from build123d import *

# Parameters (mm, degrees)
SKETCH3_W           = 114.3
SKETCH3_H           = 19.05
BOSS_EXTRUDE1_DEPTH = 3.81
SKETCH4_R           = 13.5453125
BOSS_EXTRUDE2_DEPTH = 9.525
FILLET1_R           = 2.032
SKETCH5_R           = 2.75
CUT_EXTRUDE4_DEPTH  = 12.7


with BuildPart() as part:
    # Sketch3 → Boss-Extrude1 (new body)
    with BuildSketch(Plane(origin=(0, 0, 0), x_dir=(1, 0, 0), z_dir=(0, 1, 0))):
        Rectangle(SKETCH3_W, SKETCH3_H)
    extrude(amount=BOSS_EXTRUDE1_DEPTH)

    # Sketch4 → Boss-Extrude2 (add, symmetric)
    with BuildSketch(Plane.XY):
        with BuildLine():
            Line((-36.071859255, 3.81), (36.071859255, 3.81))
            ThreePointArc((36.071859255, 3.81), (41.198342199, 6.412778013), (42.122274879, 12.087425946))
            ThreePointArc((42.122274879, 12.087425946), (41.806974837, 13.2052175), (41.567140999, 14.341594112))
            Line((41.567140999, 14.341594112), (45.319258538, 15.003193668))
            ThreePointArc((45.319258538, 15.003193668), (67.365546349, 6.979001129), (63.291557028, 30.083742702))
            ThreePointArc((63.291557028, 30.083742702), (61.010906137, 30.694841267), (58.658787305, 30.900625))
            Line((58.658787305, 30.900625), (58.658787305, 34.710625))
            ThreePointArc((58.658787305, 34.710625), (61.672505693, 34.446958806), (64.594653774, 33.663971588))
            ThreePointArc((64.594653774, 33.663971588), (75.750433611, 14.341594112), (58.658787305, 0))
            Line((58.658787305, 0), (-58.658787305, 0))
            ThreePointArc((-58.658787305, 0), (-70.930846463, 5.083253342), (-76.014099805, 17.3553125))
            ThreePointArc((-76.014099805, 17.3553125), (-55.993216901, 34.504703346), (-42.122274879, 12.087425946))
            ThreePointArc((-42.122274879, 12.087425946), (-41.198342199, 6.412778013), (-36.071859255, 3.81))
        make_face()
        with Locations(Location((-58.658787305, 17.3553125, 0), (0, 0, 180))):
            Circle(SKETCH4_R, mode=Mode.SUBTRACT)
    extrude(amount=BOSS_EXTRUDE2_DEPTH, both=True)

    # Fillet1
    # the kernel refuses this fillet: 2.032 mm, written as the material it takes off along each edge
    with BuildSketch(Plane(origin=(58.658787305, 34.710625, 0), x_dir=(0, -1, 0), z_dir=(0, 0, -1)), Plane(origin=(41.567140999, 14.341594112, 0), x_dir=(0.9848077530122078, 0.17364817766693208, 0), z_dir=(0, 0, 1))) as fillet1_piece_1:
        with BuildLine():
            CenterArc((2.16732771, -2.032), FILLET1_R, 90, 97.620348072)
            ThreePointArc((0.153273302, -2.301460275), (0.03836072, -1.153279249), (0, 0))
            Line((0, 0), (2.16732771, 0))
        make_face()
    extrude(amount=15.291396244, mode=Mode.SUBTRACT)
    with BuildSketch(Plane(origin=(58.658787305, 30.900625, 0), x_dir=(0.9978615634411592, -0.06536283505758803, 0), z_dir=(0, 0, -1)), Plane(origin=(45.319258538, 15.003193668, 0), x_dir=(0.23764666877900192, -0.9713516669148425, 0), z_dir=(0, 0, 1))) as fillet1_piece_2:
        with BuildLine():
            CenterArc((1.903537334, -2.027654697), FILLET1_R, 93.747686363, 82.504627273)
            Line((-0.124117363, -1.894837416), (0, 0))
            ThreePointArc((0, 0), (0.885360027, -0.028965791), (1.770720053, 0))
        make_face()
    extrude(amount=14.272245223, mode=Mode.SUBTRACT)
    with BuildSketch(Plane(origin=(45.319258538, 15.003193668, 0), x_dir=(-0.9848077530122076, -0.17364817766693288, 0), z_dir=(0, 0, -1)), Plane(origin=(58.658787305, 30.900625, 0), x_dir=(0, 1, 0), z_dir=(0, 0, 1))) as fillet1_piece_3:
        with BuildLine():
            CenterArc((1.898898089, -2.032), FILLET1_R, 90, 82.504627273)
            ThreePointArc((-0.115739283, -1.766933481), (-0.028965791, -0.885360027), (0, 0))
            Line((0, 0), (1.898898089, 0))
        make_face()
    extrude(amount=14.272245223, mode=Mode.SUBTRACT)
    with BuildSketch(Plane(origin=(41.567140999, 14.341594112, 0), x_dir=(0.23870589854739682, -0.9710919081110089, 0), z_dir=(0, 0, -1)), Plane(origin=(58.658787305, 34.710625, 0), x_dir=(0.9977896842762429, -0.06645107938864023, 0), z_dir=(0, 0, 1))) as fillet1_piece_4:
        with BuildLine():
            CenterArc((2.171529904, -2.027508638), FILLET1_R, 86.189825964, 97.620348072)
            Line((0.144021266, -2.162537232), (0, 0))
            ThreePointArc((0, 0), (1.153279249, 0.03836072), (2.306558498, 0))
        make_face()
    extrude(amount=15.291396244, mode=Mode.SUBTRACT)

    # Sketch5 → Cut-Extrude4 (cut)
    with BuildSketch(Plane(origin=(0, 3.81, 0), x_dir=(1, 0, 0), z_dir=(0, 1, 0))):
        with Locations(Location((-22.225, 0, 0), (0, 0, 270))):
            Circle(SKETCH5_R)
        with Locations(Location((22.225, 0, 0), (0, 0, 270))):
            Circle(SKETCH5_R)
    extrude(amount=-CUT_EXTRUDE4_DEPTH, mode=Mode.SUBTRACT)


solid = part.part
Part model, mm, in its own coordinate system. A direction names the side the tool comes from. Give positions to 0.01 mm unless a question says otherwise; leave off trailing zeros. Order: outer loops, then holes, each group sorted by start corner. A loop starts at its lowest first (then second) coordinate and runs counter-clockwise, first axis right, second up. Notation, with made-up numbers: (26, 83.5) - (41, 83.5) arc R26 cw to (41, 112.5) - close; hole circle Ø11 at (7, 7). An arc over 180 degrees is marked (long way). One line per question, with ' | ' between items.
1. Pull direction X, two halves, no side cores. Call faces 1 (the face through (75.996, 16.567, 0.133)), 2 (the face through (-1, 0, 0)), 3 (the face through (-19.5, 1.93, -0.36)): +X half, -X half, draft (parallel to the pull), parting line (faces both ways), or undercut.
Filled in:
face 1: +X half | face 2: draft | face 3: undercut
2. Band-saw the part on D-D on x = -48. List the corners of the cut face in (y, z) (3 decimals), then the cut area to 3 significant figures.
Filled in:
outline: (0, -9.525) - (8.997, -9.525) - (8.997, 9.525) - (0, 9.525) - close; (25.714, -9.525) - (31.052, -9.525) - (31.052, 9.525) - (25.714, 9.525) - close | area: 273 mm²
3. Band-saw the part on B-B on y = 6.5. List the corners of the cut face in (x, z) (1 decimal).
Filled in:
outline: (-72.2, -9.5) - (-66.8, -9.5) - (-66.8, 9.5) - (-72.2, 9.5) - close; (-50.6, -9.5) - (-41.3, -9.5) - (-41.3, 9.5) - (-50.6, 9.5) - close; (41.3, -9.5) - (50.6, -9.5) - (50.6, 9.5) - (41.3, 9.5) - close; (66.8, -9.5) - (72.2, -9.5) - (72.2, 9.5) - (66.8, 9.5) - close
4. Band-saw the part on C-C on x = -64. List the corners of the cut face in (y, z) (3 decimals), then the cut area to 3 significant figures.
Filled in:
outline: (0.842, -9.525) - (4.908, -9.525) - (4.908, 9.525) - (0.842, 9.525) - close; (29.803, -9.525) - (33.868, -9.525) - (33.868, 9.525) - (29.803, 9.525) - close | area: 155 mm²
5. Drop a flat-ended pin along its axis: P1, Ø3.5, axis at x = -22.225, z = 0, coming from the -Y side. Give the stop position or say it passes through.
Filled in:
P1: through
6. Drill centre lines: probe 1 along X at (y, z) = (16.5, -2.5); probe 2 along X at (y, z) = (1.75, 0) (3 decimals); probe 3 along X at (y, z) = (7, 0.25). Where is each one in solid material? Low to high.
Filled in:
probe 1: -75.99 to -72.18, -45.14 to -41.32, 72.18 to 75.99 | probe 2: -66.254 to -24.975, -19.475 to 19.475, 24.975 to 66.254 | probe 3: -72.59 to -67.39, -49.93 to -41.58, 41.58 to 49.93, 67.39 to 72.59
7. Which spindle directions (+Z, -Z, +X, -X, +Y, -Y) get a long thin tool onto all of the face, cutting with end or side? Do faces 4 (the face through (19.54, 1.93, -0.6)), 5 (the face through (-1, 3.81, 0)), 6 (the face through (-41.247, 6.481, 0.133)). Say none if no direction does.
Filled in:
face 4: +Y, -Y | face 5: +Z, -Z, +Y | face 6: +Z, -Z
